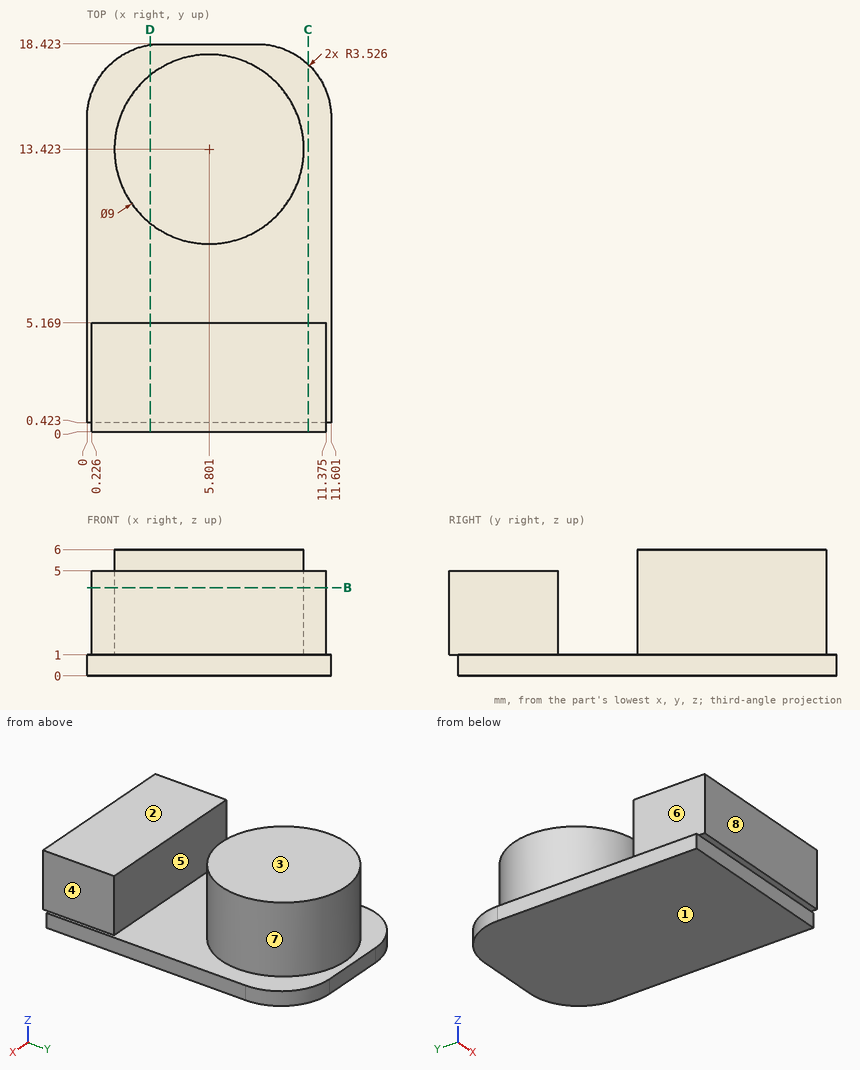
Verification items for this drawing (mm, ordinates from the low corner). A direction names the side the tool comes from. Give positions to 0.01 mm unless a question says otherwise; leave off trailing zeros. Loops run counter-clockwise (first coordinate to the right, second up) from the corner with the lowest first, then second, coordinate; pieces in that order, holes last. Notation, with made-up numbers: M 71,49 L 128,49 A23 ccw 128,76 Z; hole C -1,46 d4. An arc over 180 degrees is marked long. Write each question's results on one line, items separated by ' | '.
1) Gauge pin test, flat ends, axial feed: pin 1 (3 mm diameter, centred on y = 8.5, z = 3.5, fed in from -X); pin 2 (5.5 mm diameter, centred on x = 4.5, y = 3, fed in from +Z); pin 3 (2 mm diameter, centred on x = 5, z = 2.5, fed in from +Y); pin 4 (2 mm diameter, centred on y = 7, z = 5, fed in from -X). Record the tip position at first contact, or that the pin passes through.
Answers follow:
pin 1: x = 2.88 | pin 2: z = 5 | pin 3: y = 17.92 | pin 4: through
2) Release check for a two-part mould opening along Y. For the marked faces 6, 7 and 8 record: +Y half, -Y half, draft (parallel to the pull), parting line (faces both ways), or undercut.
Answers follow:
face 6: draft | face 7: undercut | face 8: -Y half
3) Thickness scan on line 1 (Y direction, x = 5.75, z = 4.65); line 2 (Z direction, x = 9.75, y = 1.5); line 3 (X direction, y = 13.5, z = 2.5). Record the ranges inside material, lowest first.
Answers follow:
line 1: 0 to 5.17, 8.92 to 17.92 | line 2: 0 to 5 | line 3: 1.3 to 10.3
4) Section check B-B, the plane z = 4.2. Record the boundary of the cut face in (x, y) (1 decimal), plus the area to 3 significant figures.
Answers follow:
outline: M 0.2,0 L 11.4,0 L 11.4,5.2 L 0.2,5.2 Z; C 5.8,13.4 d9 | area: 121 mm2
5) Tool access check on the marked faces 1, 2, 3, 4 and 5. Record the directions out of +Z, -Z, +X, -X, +Y, -Y that give a thin tool (end or side, any length) a straight path to the whole face; none if there is none.
Answers follow:
face 1: -Z, +X, -X, +Y, -Y | face 2: +Z, +X, -X, -Y | face 3: +Z, +X, -X, +Y, -Y | face 4: +Z, +X, +Y, -Y | face 5: +Z, +X, -X
6) Section check D-D, the plane x = 3. Record the boundary of the cut face in (y, z) (1 decimal).
Answers follow:
outline: M 0,1 L 0.4,1 L 0.4,0 L 18.4,0 L 18.4,1 L 16.9,1 L 16.9,6 L 9.9,6 L 9.9,1 L 5.2,1 L 5.2,5 L 0,5 Z
7) Section check C-C, the plane x = 10.5. Record the boundary of the cut face in (y, z).
Answers follow:
outline: M 0,1 L 0.42,1 L 0.42,0 L 17.46,0 L 17.46,1 L 5.17,1 L 5.17,5 L 0,5 Z
